Part model, mm, in its own coordinate system. A direction names the side the tool comes from. Coordinates: 2 decimals unless noted, no trailing zeros. Order: outer loops, then holes, each group sorted by start corner. A loop starts at its lowest first (then second) coordinate and runs counter-clockwise, first axis right, second up. Notation, with made-up numbers: M 30,-4 L 47,-4 A30 cw 47,35 Z; hole C 3,-26.5 d11. An arc over 180 degrees is marked long. Write item = value, one per line. Start each with the question number.
from build123d import *

# Parameters (mm, degrees)
BOSS_EXTRUDE1_DEPTH = 20
SKETCH3_W           = 19.409715081
SKETCH3_H           = 30
BOSS_EXTRUDE3_DEPTH = 15
FILLET1_R           = 2
SKETCH4_R           = 1.5
CUT_EXTRUDE1_DEPTH  = 131.530434453
FILLET2_R           = 3
SKETCH7_W           = 7.118887736
SKETCH7_H           = 19.409715081
BOSS_EXTRUDE5_DEPTH = 25
CUT_EXTRUDE3_REACH  = 126.915
SKETCH9_R           = 1.5


with BuildPart() as part:
    # Sketch1 → Boss-Extrude1 (new body)
    with BuildSketch(Plane(origin=(0, 0, 0), x_dir=(1, 0, 0), z_dir=(0, 1, 0))):
        with BuildLine():
            Line((0, -75), (0, -85))
            ThreePointArc((0, -85), (84.852300446, -5.008703332), (10, 84.409715081))
            Line((10, 84.409715081), (10, 94.409715081))
            Line((10, 94.409715081), (0, 94.409715081))
            Line((0, 94.409715081), (0, 75))
            ThreePointArc((0, 75), (75, 0), (0, -75))
        make_face()
    extrude(amount=BOSS_EXTRUDE1_DEPTH)

    # Sketch3 → Boss-Extrude3 (add)
    with BuildSketch(Plane.ZY):
        with Locations((-84.704857541, 5)):
            Rectangle(SKETCH3_W, SKETCH3_H)
    extrude(amount=BOSS_EXTRUDE3_DEPTH)

    # Fillet1
    fillet1_edges = [part.edges().sort_by_distance(p)[0] for p in [
        (84.852300446, 20, 5.008703332),
        (10, 10, -94.409715081),
        (10, 10, -84.409715081),
        (0, 10, 85),
        (0, 10, 75),
        (10, 20, -89.409715081),
        (-15, 5, -94.409715081),
        (-15, 5, -75),
        (10, 0, -89.409715081),
        (84.852300446, 0, 5.008703332),
    ]]
    fillet(fillet1_edges, radius=FILLET1_R)

    # Sketch4 → Cut-Extrude1 (cut, through all)
    with BuildSketch(Plane(origin=(0, 20, 0), x_dir=(1, 0, 0), z_dir=(0, 1, 0))):
        with Locations(Location((-7.5, 84.409715081, 0), (0, 0, 270))):
            Circle(SKETCH4_R)
        with Locations((-7.5, 94.409715081)):
            Circle(SKETCH4_R)
    extrude(amount=-CUT_EXTRUDE1_DEPTH, mode=Mode.SUBTRACT)

    # Fillet2
    # the kernel refuses this fillet: 3 mm, written as the material it takes off along each edge
    with BuildSketch(Plane(origin=(10, 17, -91.409715081), x_dir=(0, 0, -1), z_dir=(0, -1, 0))) as fillet2_piece_1:
        with BuildLine():
            CenterArc((1, -2), 2, 0, 90)
            Line((3, -2), (3, 0))
            Line((3, 0), (1, 0))
        make_face()
    revolve(axis=Axis((10, 17, -91.409715081), (1, 0, 0)), revolution_arc=90, mode=Mode.SUBTRACT)
    with BuildSketch(Plane(origin=(-20.5, 20, -94.409715081), x_dir=(0, 0, 1), z_dir=(1, 0, 0))) as fillet2_piece_2:
        with BuildLine():
            CenterArc((FILLET2_R, FILLET2_R), FILLET2_R, 180, 90)
            Line((0, FILLET2_R), (0, 0))
            Line((0, 0), (FILLET2_R, 0))
        make_face()
    extrude(amount=19, mode=Mode.SUBTRACT)
    with BuildSketch(Plane(origin=(-13.5, 20, -94.409715081), x_dir=(0, -1, 0), z_dir=(1, 0, 0))) as fillet2_piece_3:
        with BuildLine():
            CenterArc((FILLET2_R, -FILLET2_R), FILLET2_R, 90, 90)
            Line((0, -FILLET2_R), (0, 0))
            Line((0, 0), (FILLET2_R, 0))
        make_face()
    extrude(amount=23.5, mode=Mode.SUBTRACT)

    # Sketch7 → Boss-Extrude5 (add)
    with BuildSketch(Plane(origin=(0, 0, 0), x_dir=(-1, 0, 0), z_dir=(0, -1, 0))):
        with Locations((-3.559443868, 84.704857541)):
            Rectangle(SKETCH7_W, SKETCH7_H)
    extrude(amount=BOSS_EXTRUDE5_DEPTH)

    # Sketch9 → Cut-Extrude3 (cut, up to next)
    with BuildSketch(Plane(origin=(7.118887736, 0, 0), x_dir=(0, 0, -1), z_dir=(1, 0, 0)), mode=Mode.PRIVATE) as cut_extrude3_sk1:
        with Locations((84.70485754, -17.5)):
            Circle(SKETCH9_R)
    cut_extrude3_tool1 = extrude(cut_extrude3_sk1.sketch, amount=-CUT_EXTRUDE3_REACH, mode=Mode.PRIVATE) & part.part
    add(cut_extrude3_tool1.solids().sort_by_distance((7.118888, -17.5, -84.704858))[0], mode=Mode.SUBTRACT)


solid = part.part
Item 1: 3-axis set-ups, long thin cutter, end or side, ignore diameter. For faces 1 (the flat face through (-15, 5, -85)), 2 (the flat face through (7.119, -12, -85)), 3 (the flat face through (0, 10, 80)), 4 (the flat face through (10, 10, -89)), 5 (the flat face through (0, -15.7, -84.6)): which of +Z, -Z, +X, -X, +Y, -Y reach the whole face in a straight line?
Item 2: Cut at C-C, the plane y = -13. Write the cut outline in (x, z).
Item 3: Flat gauge pins, fed straight in: pin 1 (12 mm diameter, centred on y = 4.5, z = 53, fed in from +X); pin 2 (15.5 mm diameter, centred on y = -18, z = -85.5, fed in from +X); pin 3 (4 mm diameter, centred on y = -17.5, z = -84.7, fed in from -X); pin 4 (16.5 mm diameter, centred on y = -18, z = -85, fed in from -X). Where does each tip first touch, or does it go through?
Item 4: Pull direction Z, two halves, no side cores. Call faces 6 (the flat face through (74, 20, -18)), 7 (the flat face through (1, 1, -94.41)), 8 (the cylindrical face through (74.955, 9.86, -2.609)): pulls with the +Z half, pulls with the -Z half, needs draft (parallel to the pull), parting line crosses it, or undercut.
Item 5: Cut at B-B, the plane y = -2. Write the cut outline in (x, z), and give its area (3 significant figures).
Item 6: Wall check: line 1 along Y through (x, z) = (54.5, -56.5); line 2 along Z through (x, y) = (25.5, 0.5); line 3 along X through (y, z) = (3, 3). Give the ranges that are in metal, low to high. Write a range as [from, to].
Filled sheet:
q1.face_1 = +Z, -Z, -X, +Y, -Y
q1.face_2 = +Z, -Z, +X, -Y
q1.face_3 = +Z, -X, +Y, -Y
q1.face_4 = -Z, +X, +Y, -Y
q1.face_5 = +Z, -Z, -X, -Y
q2.outline = M 0,-94.41 L 7.12,-94.41 L 7.12,-75 L 0,-75 Z
q3.pin_1 = 70.82
q3.pin_2 = 7.12
q3.pin_3 = 0
q3.pin_4 = -15
q4.face_6 = needs draft
q4.face_7 = pulls with the -Z half
q4.face_8 = undercut
q5.outline = M -15,-92.41 A2 ccw -13,-94.41 L -9,-94.41 A1.5 cw -6,-94.41 L 7.12,-94.41 L 7.12,-75 L -13,-75 A2 ccw -15,-77 Z; hole C -7.5,-84.41 d3
q5.area = 417 mm2
q6.line_1 = [0, 20]
q6.line_2 = [-80.37, -70.53], [70.53, 80.37]
q6.line_3 = [74.94, 84.95]
